from build123d import *

# Parameters (mm, degrees)
F0_R     = 7.5
F1_DEPTH = 25


with BuildPart() as f1:
    # F0 (on Front) → F1 (new body)
    with BuildSketch(Plane.XZ):
        with BuildLine():
            Line((3, 24.819347), (3, 29.849623))
            ThreePointArc((3, 29.849623), (0, 30), (-3, 29.849623))
            Line((-3, 29.849623), (-3, 24.819347))
            ThreePointArc((-3, 24.819347), (-4.877258, 24.519632), (-6.726314, 24.078137))
            ThreePointArc((-6.726314, 24.078137), (-9.567086, 23.096988), (-12.269592, 21.782037))
            ThreePointArc((-12.269592, 21.782037), (-13.889256, 20.78674), (-15.428608, 19.671249))
            ThreePointArc((-15.428608, 19.671249), (-17.67767, 17.67767), (-19.671249, 15.428608))
            ThreePointArc((-19.671249, 15.428608), (-20.78674, 13.889256), (-21.782037, 12.269592))
            ThreePointArc((-21.782037, 12.269592), (-23.096988, 9.567086), (-24.078137, 6.726314))
            ThreePointArc((-24.078137, 6.726314), (-24.519632, 4.877258), (-24.819347, 3))
            ThreePointArc((-24.819347, 3), (-25, 0), (-24.819347, -3))
            ThreePointArc((-24.819347, -3), (-24.519632, -4.877258), (-24.078137, -6.726314))
            ThreePointArc((-24.078137, -6.726314), (-23.096988, -9.567086), (-21.782037, -12.269592))
            ThreePointArc((-21.782037, -12.269592), (-20.78674, -13.889256), (-19.671249, -15.428608))
            ThreePointArc((-19.671249, -15.428608), (-17.67767, -17.67767), (-15.428608, -19.671249))
            ThreePointArc((-15.428608, -19.671249), (-13.889256, -20.78674), (-12.269592, -21.782037))
            ThreePointArc((-12.269592, -21.782037), (-9.567086, -23.096988), (-6.726314, -24.078137))
            ThreePointArc((-6.726314, -24.078137), (-4.877258, -24.519632), (-3, -24.819347))
            ThreePointArc((-3, -24.819347), (0, -25), (3, -24.819347))
            ThreePointArc((3, -24.819347), (4.877258, -24.519632), (6.726314, -24.078137))
            ThreePointArc((6.726314, -24.078137), (9.567086, -23.096988), (12.269592, -21.782037))
            ThreePointArc((12.269592, -21.782037), (13.889256, -20.78674), (15.428608, -19.671249))
            ThreePointArc((15.428608, -19.671249), (17.67767, -17.67767), (19.671249, -15.428608))
            ThreePointArc((19.671249, -15.428608), (20.78674, -13.889256), (21.782037, -12.269592))
            ThreePointArc((21.782037, -12.269592), (23.096988, -9.567086), (24.078137, -6.726314))
            ThreePointArc((24.078137, -6.726314), (24.519632, -4.877258), (24.819347, -3))
            ThreePointArc((24.819347, -3), (25, 0), (24.819347, 3))
            ThreePointArc((24.819347, 3), (24.519632, 4.877258), (24.078137, 6.726314))
            ThreePointArc((24.078137, 6.726314), (23.096988, 9.567086), (21.782037, 12.269592))
            ThreePointArc((21.782037, 12.269592), (20.78674, 13.889256), (19.671249, 15.428608))
            ThreePointArc((19.671249, 15.428608), (17.67767, 17.67767), (15.428608, 19.671249))
            ThreePointArc((15.428608, 19.671249), (13.889256, 20.78674), (12.269592, 21.782037))
            ThreePointArc((12.269592, 21.782037), (9.567086, 23.096988), (6.726314, 24.078137))
            ThreePointArc((6.726314, 24.078137), (4.877258, 24.519632), (3, 24.819347))
        make_face()
        Circle(F0_R, mode=Mode.SUBTRACT)
        with BuildLine():
            Line((8.651318, 28.725506), (6.726314, 24.078137))
            ThreePointArc((6.726314, 24.078137), (9.567086, 23.096988), (12.269592, 21.782037))
            Line((12.269592, 21.782037), (14.194595, 26.429406))
            ThreePointArc((14.194595, 26.429406), (11.480503, 27.716386), (8.651318, 28.725506))
        make_face()
        with BuildLine():
            ThreePointArc((-12.269592, 21.782037), (-9.567086, 23.096988), (-6.726314, 24.078137))
            Line((-6.726314, 24.078137), (-8.651318, 28.725506))
            ThreePointArc((-8.651318, 28.725506), (-11.480503, 27.716386), (-14.194595, 26.429406))
            Line((-14.194595, 26.429406), (-12.269592, 21.782037))
        make_face()
        with BuildLine():
            Line((18.985551, 23.228191), (15.428608, 19.671249))
            ThreePointArc((15.428608, 19.671249), (17.67767, 17.67767), (19.671249, 15.428608))
            Line((19.671249, 15.428608), (23.228191, 18.985551))
            ThreePointArc((23.228191, 18.985551), (21.213203, 21.213203), (18.985551, 23.228191))
        make_face()
        with BuildLine():
            ThreePointArc((-19.671249, 15.428608), (-17.67767, 17.67767), (-15.428608, 19.671249))
            Line((-15.428608, 19.671249), (-18.985551, 23.228191))
            ThreePointArc((-18.985551, 23.228191), (-21.213203, 21.213203), (-23.228191, 18.985551))
            Line((-23.228191, 18.985551), (-19.671249, 15.428608))
        make_face()
        with BuildLine():
            Line((26.429406, 14.194595), (21.782037, 12.269592))
            ThreePointArc((21.782037, 12.269592), (23.096988, 9.567086), (24.078137, 6.726314))
            Line((24.078137, 6.726314), (28.725506, 8.651318))
            ThreePointArc((28.725506, 8.651318), (27.716386, 11.480503), (26.429406, 14.194595))
        make_face()
        with BuildLine():
            ThreePointArc((-24.078137, 6.726314), (-23.096988, 9.567086), (-21.782037, 12.269592))
            Line((-21.782037, 12.269592), (-26.429406, 14.194595))
            ThreePointArc((-26.429406, 14.194595), (-27.716386, 11.480503), (-28.725506, 8.651318))
            Line((-28.725506, 8.651318), (-24.078137, 6.726314))
        make_face()
        with BuildLine():
            Line((29.849623, 3), (24.819347, 3))
            ThreePointArc((24.819347, 3), (25, 0), (24.819347, -3))
            Line((24.819347, -3), (29.849623, -3))
            ThreePointArc((29.849623, -3), (30, 0), (29.849623, 3))
        make_face()
        with BuildLine():
            ThreePointArc((-24.819347, -3), (-25, 0), (-24.819347, 3))
            Line((-24.819347, 3), (-29.849623, 3))
            ThreePointArc((-29.849623, 3), (-30, 0), (-29.849623, -3))
            Line((-29.849623, -3), (-24.819347, -3))
        make_face()
        with BuildLine():
            Line((28.725506, -8.651318), (24.078137, -6.726314))
            ThreePointArc((24.078137, -6.726314), (23.096988, -9.567086), (21.782037, -12.269592))
            Line((21.782037, -12.269592), (26.429406, -14.194595))
            ThreePointArc((26.429406, -14.194595), (27.716386, -11.480503), (28.725506, -8.651318))
        make_face()
        with BuildLine():
            ThreePointArc((-21.782037, -12.269592), (-23.096988, -9.567086), (-24.078137, -6.726314))
            Line((-24.078137, -6.726314), (-28.725506, -8.651318))
            ThreePointArc((-28.725506, -8.651318), (-27.716386, -11.480503), (-26.429406, -14.194595))
            Line((-26.429406, -14.194595), (-21.782037, -12.269592))
        make_face()
        with BuildLine():
            Line((23.228191, -18.985551), (19.671249, -15.428608))
            ThreePointArc((19.671249, -15.428608), (17.67767, -17.67767), (15.428608, -19.671249))
            Line((15.428608, -19.671249), (18.985551, -23.228191))
            ThreePointArc((18.985551, -23.228191), (21.213203, -21.213203), (23.228191, -18.985551))
        make_face()
        with BuildLine():
            ThreePointArc((-15.428608, -19.671249), (-17.67767, -17.67767), (-19.671249, -15.428608))
            Line((-19.671249, -15.428608), (-23.228191, -18.985551))
            ThreePointArc((-23.228191, -18.985551), (-21.213203, -21.213203), (-18.985551, -23.228191))
            Line((-18.985551, -23.228191), (-15.428608, -19.671249))
        make_face()
        with BuildLine():
            Line((14.194595, -26.429406), (12.269592, -21.782037))
            ThreePointArc((12.269592, -21.782037), (9.567086, -23.096988), (6.726314, -24.078137))
            Line((6.726314, -24.078137), (8.651318, -28.725506))
            ThreePointArc((8.651318, -28.725506), (11.480503, -27.716386), (14.194595, -26.429406))
        make_face()
        with BuildLine():
            ThreePointArc((-6.726314, -24.078137), (-9.567086, -23.096988), (-12.269592, -21.782037))
            Line((-12.269592, -21.782037), (-14.194595, -26.429406))
            ThreePointArc((-14.194595, -26.429406), (-11.480503, -27.716386), (-8.651318, -28.725506))
            Line((-8.651318, -28.725506), (-6.726314, -24.078137))
        make_face()
        with BuildLine():
            Line((3, -29.849623), (3, -24.819347))
            ThreePointArc((3, -24.819347), (0, -25), (-3, -24.819347))
            Line((-3, -24.819347), (-3, -29.849623))
            ThreePointArc((-3, -29.849623), (0, -30), (3, -29.849623))
        make_face()
    extrude(amount=F1_DEPTH)


solid = f1.part
Geometry check sheet. Reference: the model listing, model coordinates, mm. A direction names the side the tool comes from. Round coordinates to 2 decimals unless told otherwise and drop trailing zeros. Loops run counter-clockwise (first coordinate to the right, second up) from the corner with the lowest first, then second, coordinate; pieces in that order, holes last. Notation, with made-up numbers: (86.5, 77.25) -> (135.5, 77.25) arc R18 cw to (135.5, 100.25) -> close; hole circle Ø1 at (-6, -10). An arc over 180 degrees is marked (long way). Answer as a JSON object with one key per item and string values. Group by question number.
Item 1: Cross-section at D-D, the plane x = 17.5. Record the cut outline in (y, z), plus the area to 3 significant figures.
Item 2: Cross-section at A-A, the plane z = 0. Record the cut outline in (x, y).
Item 3: Cross-section at C-C, the plane z = -9.5. Record the cut outline in (x, y), plus the area to 3 significant figures.
Item 4: Set-up check for faces 1 (the face through (26.43, -12.32, -7.7)), 2 (the face through (0, -12, 30)), 3 (the face through (-13.246, -12.325, 24.138)), 4 (the face through (3, -12, -27)), 5 (the face through (-27, -12, 3)): record each of +Z, -Z, +X, -X, +Y, -Y from which the full face is reachable in a straight line by a thin tool's end or side.
Item 5: Cross-section at B-B, the plane x = 0. Record the cut outline in (y, z).
Item 6: Depth check by flat-ended pin: pin 1 Ø1.5 at (x, y) = (-21, -21) entering from -Z; pin 2 Ø4 at (x, y) = (-12.5, -21.5) entering from -Z; pin 3 Ø6 at (y, z) = (-5, -23.5) entering from +X; pin 4 Ø13.5 at (x, z) = (0, 0) entering from +Y. Enter the tip coordinate at first touch or a pass-through.
Item 7: Release check for a two-part mould opening along X. For faces 6 (the face through (24.525, -12.325, 4.851)), 7 (the face through (-26.369, -12.325, -7.675)), 8 (the face through (13.87, -12.32, -20.8)) record: pulls with the +X half, pulls with the -X half, needs draft (parallel to the pull), parting line crosses it, or undercut.
Item 8: Thickness scan on line 1 along Z through (x, y) = (0, -9.75); line 2 along X through (y, z) = (-23.25, 13); line 3 along X through (y, z) = (-19.25, 1.5). Record the ranges inside material, lowest first.
Determined:
{
 "1": {"outline": "(-25, -21.74) -> (0, -21.74) -> (0, 21.74) -> (-25, 21.74) -> close", "area": "1,090 mm²"},
 "2": {"outline": "(-30, -25) -> (-7.5, -25) -> (-7.5, 0) -> (-30, 0) -> close; (7.5, -25) -> (30, -25) -> (30, 0) -> (7.5, 0) -> close"},
 "3": {"outline": "(-28.46, -25) -> (28.46, -25) -> (28.46, 0) -> (-28.46, 0) -> close", "area": "1,420 mm²"},
 "4": {"face 1": "+X, +Y, -Y", "face 2": "+Z, +Y, -Y", "face 3": "+Y, -Y", "face 4": "-Z, +Y, -Y", "face 5": "-X, +Y, -Y"},
 "5": {"outline": "(-25, -30) -> (0, -30) -> (0, -7.5) -> (-25, -7.5) -> close; (-25, 7.5) -> (0, 7.5) -> (0, 30) -> (-25, 30) -> close"},
 "6": {"pin 1": "stops at z = -22.13", "pin 2": "stops at z = -28.1", "pin 3": "stops at x = 21.9", "pin 4": "passes through"},
 "7": {"face 6": "pulls with the +X half", "face 7": "pulls with the -X half", "face 8": "undercut"},
 "8": {"line 1": "z = -30 to -7.5, 7.5 to 30", "line 2": "x = -27.04 to -23.55, -21.35 to 21.35, 23.55 to 27.04", "line 3": "x = -29.96 to -7.35, 7.35 to 29.96"}
}
